Source: three-view drawing plus pictorial views. Frame: mm from the lowest corner of the part. A direction names the side the tool comes from. Give positions to 0.01 mm unless a question says otherwise; leave off trailing zeros. Write each loop counter-clockwise with the first axis right and the second up, starting at its lowest first coordinate (ties: lowest second). Pieces come first, ordered by that corner, then holes.
Q1. Reachability of the marked faces 1 and 2 from +Z, -Z, +X, -X, +Y, -Y: full face, straight path, thin tool, end or side. Return the list, or none.
Q2. Cut plane C-C on x = 105. Return the cut outline in (y, z), plus the area to 3 significant figures.
Q3. Cut plane A-A on z = 7. Return the cut outline in (x, y).
Q4. Line query: L1, parallel to Y at x = 74.5, z = 18.25; L2, parallel to Z at x = 95.5, y = 17. Output: solid intervals per line, ascending.
Q5. Pin query (flat end, axial travel): pin 1 (6.5 mm diameter, centred on x = 77.4, y = 28.39, fed in from +Z). Return the tip coordinate at first contact, or that it passes through.
Q6. Draft query along Z for the marked faces 3, 4 and 5. Return one class per face: pulls with the +Z half, pulls with the -Z half, needs draft (parallel to the pull), parting line crosses it, or undercut.
Q7. Cut plane B-B on y = 12.5. Return the cut outline in (x, z).
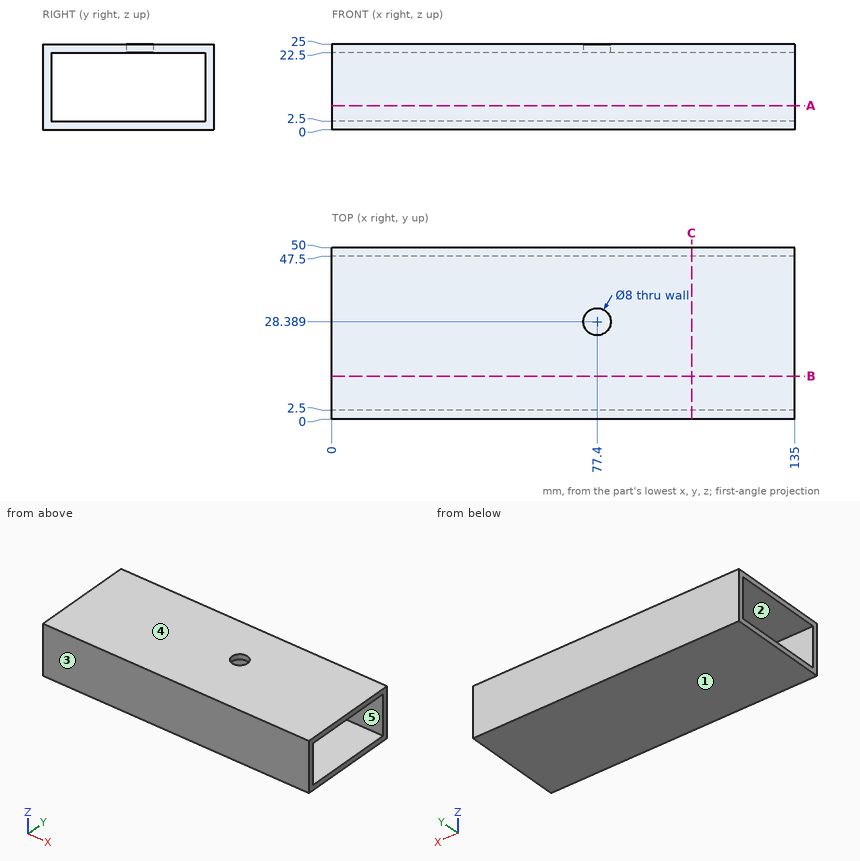
Data:
1. face 1: -Z, +X, -X, +Y, -Y
1. face 2: +X, -X
2. outline: (0, 0) - (50, 0) - (50, 25) - (0, 25) - close; hole (2.5, 2.5) - (47.5, 2.5) - (47.5, 22.5) - (2.5, 22.5) - close
2. area: 350 mm2
3. outline: (0, 0) - (135, 0) - (135, 2.5) - (0, 2.5) - close; (0, 47.5) - (135, 47.5) - (135, 50) - (0, 50) - close
4. L1: y = 0 to 2.5, 47.5 to 50
4. L2: z = 0 to 2.5, 22.5 to 25
5. pin 1: stops at z = 2.5
6. face 3: needs draft
6. face 4: pulls with the +Z half
6. face 5: undercut
7. outline: (0, 0) - (135, 0) - (135, 2.5) - (0, 2.5) - close; (0, 22.5) - (135, 22.5) - (135, 25) - (0, 25) - close
